from build123d import *

# Parameters (mm, degrees)
SKETCH1_W             = 1
SKETCH1_H             = 25.4
SKETCH1_W_2           = 13.7
SKETCH1_H_2           = 1
BOSS_EXTRUDE1_DEPTH   = 63.5
SKETCH2_W             = 20.32
SKETCH2_H             = 40.64
CUT_EXTRUDE1_DEPTH    = 70.932109935
F_5_0MM_DOWEL_HOLE1_D = 5


with BuildPart() as part:
    # Sketch1 → Boss-Extrude1 (new body)
    with BuildSketch(Plane(origin=(0, 0, 0), x_dir=(1, 0, 0), z_dir=(0, 1, 0))):
        with Locations((13.2, 13.7)):
            Rectangle(SKETCH1_W, SKETCH1_H)
        with Locations((6.85, 0.5)):
            Rectangle(SKETCH1_W_2, SKETCH1_H_2)
    extrude(amount=BOSS_EXTRUDE1_DEPTH)

    # Sketch2 → Cut-Extrude1 (cut, through all)
    with BuildSketch(Plane.ZY.offset(-12.7)):
        with Locations((-13.7, 31.75)):
            Rectangle(SKETCH2_W, SKETCH2_H)
    extrude(amount=-CUT_EXTRUDE1_DEPTH, mode=Mode.SUBTRACT)

    # Ø5.0mm Dowel Hole1 (through all)
    with Locations(Plane.ZY.offset(-12.7)):
        with Locations((-9.2, 6.6), (-18.2, 56.9), (-9.2, 56.9), (-18.2, 6.6)):
            Hole(F_5_0MM_DOWEL_HOLE1_D / 2)


solid = part.part
Read the model definition and answer for the solid it produces. Units are mm, in the model's axes. A direction names the side the tool comes from. Round coordinates to 2 decimals unless told otherwise and drop trailing zeros. Loops run counter-clockwise (first coordinate to the right, second up) from the corner with the lowest first, then second, coordinate; pieces in that order, holes last. Notation, with made-up numbers: (10, 8) - (18, 8) arc R24 cw to (18, 23) - close; hole circle Ø5 at (88, 30). An arc over 180 degrees is marked (long way). One line per question, with ' | ' between items. Start each with the question number.
Q1. For faces 4 (the flat face through (12.7, 31, -25)), 5 (the flat face through (13, 0, -9)), determine the directions among +Z, -Z, +X, -X, +Y, -Y from which every point of the face is accessible in a straight line to the end or side of a thin tool.
Q2. Find the intervals of material crossed by L1, parallel to Y at x = 13.45, z = -9.2; L2, parallel to Z at x = 7.25, y = 28; L3, parallel to X at y = 60, z = -11.5, in increasing order.
Q3. For a pull along Z with two mould halves and no side action, classify faces 1 (the flat face through (13.7, 31, -1)), 2 (the cylindrical face through (13.21, 54.46, -8.66)), 3 (the flat face through (6, 31, -1)) as +Z half, -Z half, draft (parallel to the pull), parting line (faces both ways), or undercut.
Q4. Section B-B on z = -17.5 is taken. Give the vertices of the cut face in (x, y).
Q5. Section D-D on y = 19 is taken. Give the vertices of the cut face in (x, z).
Q6. Flat-ended cylindrical pins translate along their axes: pin 1 (4.5 mm diameter, centred on y = 6.6, z = -18.2, fed in from +X); pin 2 (2 mm diameter, centred on y = 30, z = -3.5, fed in from -X); pin 3 (6 mm diameter, centred on x = 7, y = 43.5, fed in from -Z). Find the tip coordinate at first contact, or state that the pin passes through.
Q7. Section C-C on y = 56.9 is taken. Give the vertices of the cut face in (x, z).
Q8. Section A-A on z = -4.5 is taken. Give the vertices of the cut face in (x, y).
Established:
1) face 4: -Z, -X, +Y, -Y | face 5: +Z, -Z, +X, -X, -Y
2) L1: 0 to 4.1, 9.1 to 11.43, 52.07 to 54.4, 59.4 to 63.5 | L2: -1 to 0 | L3: 12.7 to 13.7
3) face 1: draft | face 2: undercut | face 3: -Z half
4) outline: (12.7, 0) - (13.7, 0) - (13.7, 4.2) - (12.7, 4.2) - close; (12.7, 9) - (13.7, 9) - (13.7, 11.43) - (12.7, 11.43) - close; (12.7, 52.07) - (13.7, 52.07) - (13.7, 54.5) - (12.7, 54.5) - close; (12.7, 59.3) - (13.7, 59.3) - (13.7, 63.5) - (12.7, 63.5) - close
5) outline: (0, -1) - (12.7, -1) - (12.7, -3.54) - (13.7, -3.54) - (13.7, 0) - (0, 0) - close; (12.7, -26.4) - (13.7, -26.4) - (13.7, -23.86) - (12.7, -23.86) - close
6) pin 1: through | pin 2: x = 12.7 | pin 3: z = -1
7) outline: (0, -1) - (12.7, -1) - (12.7, -6.7) - (13.7, -6.7) - (13.7, 0) - (0, 0) - close; (12.7, -26.4) - (13.7, -26.4) - (13.7, -20.7) - (12.7, -20.7) - close; (12.7, -15.7) - (13.7, -15.7) - (13.7, -11.7) - (12.7, -11.7) - close
8) outline: (12.7, 0) - (13.7, 0) - (13.7, 11.43) - (12.7, 11.43) - close; (12.7, 52.07) - (13.7, 52.07) - (13.7, 63.5) - (12.7, 63.5) - close
